from build123d import *

# Parameters (mm, degrees)
SKETCH1_R           = 37.5
SKETCH1_R_2         = 17.5
BOSS_EXTRUDE1_DEPTH = 76
SKETCH1_3_R         = 17.5
BOSS_EXTRUDE2_DEPTH = 78
SKETCH1_4_R         = 39
SKETCH1_4_R_2       = 37.5
BOSS_EXTRUDE3_DEPTH = 32
SKETCH2_R           = 1.75
CUT_EXTRUDE1_DEPTH  = 7
FILLET1_R           = 0.5
CHAMFER1_SIZE       = 0.5
CHAMFER2_SIZE       = 21.5
CHAMFER2_SIZE2      = 20
CHAMFER3_SIZE       = 1
SKETCH4_R           = 4
CUT_EXTRUDE2_DEPTH  = 68


with BuildPart() as part:
    # Sketch1 → Boss-Extrude1 (new body)
    with BuildSketch(Plane(origin=(0, 0, 0), x_dir=(1, 0, 0), z_dir=(0, 1, 0))):
        with Locations(Location((0, 0, 0), (0, 0, 270))):
            Circle(SKETCH1_R)
        with Locations(Location((0, 0, 0), (0, 0, 270))):
            Circle(SKETCH1_R_2, mode=Mode.SUBTRACT)
    extrude(amount=BOSS_EXTRUDE1_DEPTH)

    # Sketch1<3> → Boss-Extrude2 (add)
    with BuildSketch(Plane(origin=(0, 0, 0), x_dir=(1, 0, 0), z_dir=(0, 1, 0))):
        with Locations(Location((0, 0, 0), (0, 0, 270))):
            Circle(SKETCH1_3_R)
    extrude(amount=BOSS_EXTRUDE2_DEPTH)

    # Sketch1<4> → Boss-Extrude3 (add)
    with BuildSketch(Plane(origin=(0, 0, 0), x_dir=(1, 0, 0), z_dir=(0, 1, 0))):
        with Locations(Location((0, 0, 0), (0, 0, 270))):
            Circle(SKETCH1_4_R)
        with Locations(Location((0, 0, 0), (0, 0, 270))):
            Circle(SKETCH1_4_R_2, mode=Mode.SUBTRACT)
    extrude(amount=BOSS_EXTRUDE3_DEPTH)

    # Sketch2 → Cut-Extrude1 (cut)
    with BuildSketch(Plane(origin=(0, 76, 0), x_dir=(1, 0, 0), z_dir=(0, 1, 0))):
        with Locations(Location((0, 27.5, 0), (0, 0, 270))):
            Circle(SKETCH2_R)
        with Locations(Location((26.154054198, 8.497967345, 0), (0, 0, 270))):
            Circle(SKETCH2_R)
        with Locations(Location((16.164094438, -22.247967345, 0), (0, 0, 270))):
            Circle(SKETCH2_R)
        with Locations(Location((-16.164094438, -22.247967345, 0), (0, 0, 270))):
            Circle(SKETCH2_R)
        with Locations(Location((-26.154054198, 8.497967345, 0), (0, 0, 270))):
            Circle(SKETCH2_R)
    extrude(amount=-CUT_EXTRUDE1_DEPTH, mode=Mode.SUBTRACT)

    # Fillet1
    fillet1_edges = [part.edges().sort_by_distance(p)[0] for p in [
        (0, 32, -39),
    ]]
    fillet(fillet1_edges, radius=FILLET1_R)

    # Chamfer1
    chamfer1_edges = [part.edges().sort_by_distance(p)[0] for p in [
        (0, 76, -37.5),
    ]]
    chamfer(chamfer1_edges, length=CHAMFER1_SIZE)

    # Chamfer2
    chamfer2_edges = [part.edges().sort_by_distance(p)[0] for p in [
        (0, 0, -39),
    ]]
    chamfer2_side = [part.faces().sort_by_distance(p)[0] for p in [
        (0, 0, 0),
    ]]
    chamfer(chamfer2_edges, length=CHAMFER2_SIZE, length2=CHAMFER2_SIZE2, reference=chamfer2_side[0])

    # Chamfer3
    chamfer3_edges = [part.edges().sort_by_distance(p)[0] for p in [
        (0, 78, -17.5),
    ]]
    chamfer(chamfer3_edges, length=CHAMFER3_SIZE)

    # Sketch4 → Cut-Extrude2 (cut)
    with BuildSketch(Plane.XZ):
        with Locations(Location((0, 0, 0), (0, 0, 270))):
            Circle(SKETCH4_R)
    extrude(amount=-CUT_EXTRUDE2_DEPTH, mode=Mode.SUBTRACT)


solid = part.part
Read the model definition and answer for the solid it produces. Units are mm, in the model's axes. A direction names the side the tool comes from. Coordinates: 2 decimals unless noted, no trailing zeros. Loops run counter-clockwise (first coordinate to the right, second up) from the corner with the lowest first, then second, coordinate; pieces in that order, holes last. Notation, with made-up numbers: (55.5, 37.5) -> (89.5, 37.5) arc R21 cw to (89.5, 60.5) -> close; hole circle Ø5 at (-21.5, 40.5). An arc over 180 degrees is marked (long way). Answer in a Markdown table with one row per item.
Item 1: For a pull along Z with two mould halves and no side action, classify faces 1 (the flat face through (-26, 69, -9)), 2 (the flat face through (0, 78, 0)), 3 (the cylindrical face through (-10.648, 76.493, -13.887)) as released by +Z, released by -Z, zero draft, split by the parting line, or undercut.
Returned:
| item | result |
|---|---|
| face 1 | undercut |
| face 2 | zero draft |
| face 3 | split by the parting line |
Item 2: Straight lines are drawn through the part: line 1 along X through (y, z) = (4, -1.5); line 2 along X through (y, z) = (75, 1); line 3 along Z through (x, y) = (2, 23.5). For each, find the intervals that lie inside material, in ascending order. Write a range as [from, to].
Returned:
| item | result |
|---|---|
| line 1 | x = [-21.75, -3.71], [3.71, 21.75] |
| line 2 | x = [-37.49, 37.49] |
| line 3 | z = [-38.95, -3.46], [3.46, 38.95] |
Item 3: A cutting plane is placed at D-D on y = 22. Determine the outline of the cut face in (x, z), plus the area to 3 significant figures.
Returned:
| item | result |
|---|---|
| outline | circle Ø78 at (0, 0); hole circle Ø8 at (0, 0) |
| area | 4,730 mm^2 |
Item 4: A cutting plane is placed at C-C on y = 37. Determine the outline of the cut face in (x, z), plus the area to 3 significant figures.
Returned:
| item | result |
|---|---|
| outline | circle Ø75 at (0, 0); hole circle Ø8 at (0, 0) |
| area | 4,370 mm^2 |
Item 5: A cutting plane is placed at A-A on x = 0. Determine the outline of the cut face in (y, z), plus the area to 3 significant figures.
Returned:
| item | result |
|---|---|
| outline | (0, -17.5) -> (20, -39) -> (31.5, -39) arc R0.5 ccw to (32, -38.5) -> (32, -37.5) -> (75.5, -37.5) -> (76, -37) -> (76, -29.25) -> (69, -29.25) -> (69, -25.75) -> (76, -25.75) -> (76, -17.5) -> (77, -17.5) -> (78, -16.5) -> (78, 16.5) -> (77, 17.5) -> (76, 17.5) -> (76, 37) -> (75.5, 37.5) -> (32, 37.5) -> (32, 38.5) arc R0.5 ccw to (31.5, 39) -> (20, 39) -> (0, 17.5) -> (0, 4) -> (68, 4) -> (68, -4) -> (0, -4) -> close |
| area | 4,870 mm^2 |
Item 6: For faces 4 (the cylindrical face through (-22.818, 53.445, -29.759)), 5 (the cylindrical face through (38.668, 25.67, -5.077)), 6 (the cylindrical face through (-3.905, 33.524, 0.867)), determine the directions among +Z, -Z, +X, -X, +Y, -Y from which every point of the face is accessible in a straight line to the end or side of a thin tool.
Returned:
| item | result |
|---|---|
| face 4 | +Y |
| face 5 | +Y, -Y |
| face 6 | -Y |
Item 7: A cutting plane is placed at B-B on z = 0. Determine the outline of the cut face in (x, y), plus the area to 3 significant figures.
Returned:
| item | result |
|---|---|
| outline | (-39, 20) -> (-17.5, 0) -> (-4, 0) -> (-4, 68) -> (4, 68) -> (4, 0) -> (17.5, 0) -> (39, 20) -> (39, 31.5) arc R0.5 ccw to (38.5, 32) -> (37.5, 32) -> (37.5, 75.5) -> (37, 76) -> (17.5, 76) -> (17.5, 77) -> (16.5, 78) -> (-16.5, 78) -> (-17.5, 77) -> (-17.5, 76) -> (-37, 76) -> (-37.5, 75.5) -> (-37.5, 32) -> (-38.5, 32) arc R0.5 ccw to (-39, 31.5) -> close |
| area | 4,890 mm^2 |
Item 8: Each of these flat-tipped pins is pushed along its axis until it touches: P1, Ø3, axis at x = -16.16, z = 22.25, coming from the -Y side; P2, Ø1, axis at x = 26.5, z = -8.5, coming from the +Y side; P3, Ø4, axis at x = -15.5, z = 22.5, coming from the +Y side. Where does it stop, or does it pass through?
Returned:
| item | result |
|---|---|
| P1 | stops at y = 7.91 |
| P2 | stops at y = 69 |
| P3 | stops at y = 76 |
